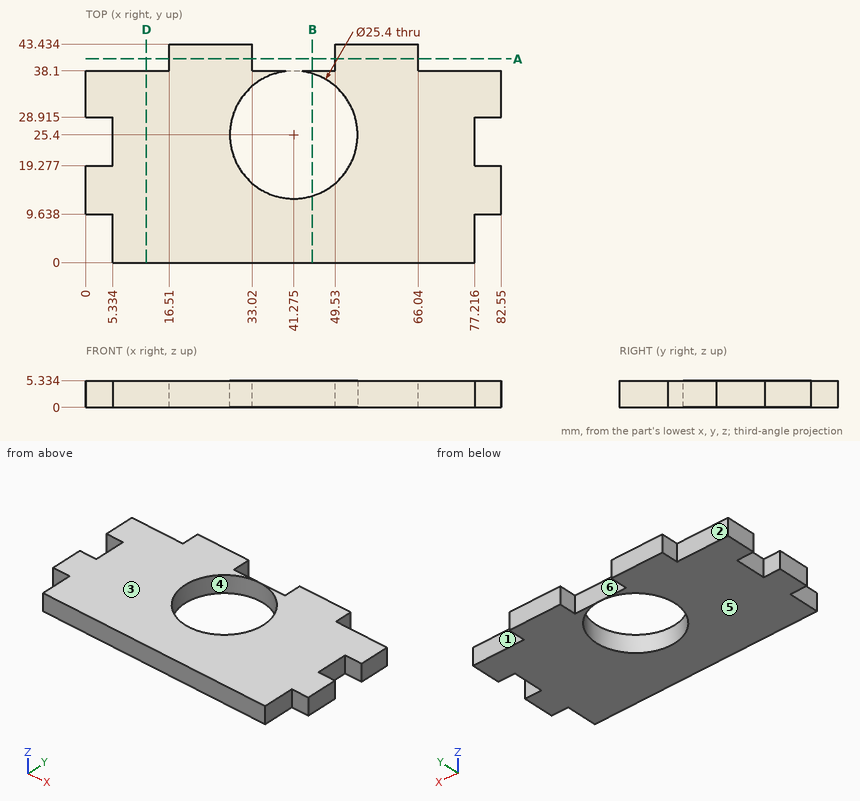
Job drawing, mm, ordinate dimensions from the low corner. One solid piece. A direction names the side the tool comes from. Coordinates: 2 decimals unless noted, no trailing zeros. Order: outer loops, then holes, each group sorted by start corner. A loop starts at its lowest first (then second) coordinate and runs counter-clockwise, first axis right, second up. Notation, with made-up numbers: M 69,87.25 L 92,87.25 A11 ccw 92,107.25 Z; hole C 89.5,10.5 d10. An arc over 180 degrees is marked long. Return JSON: item names as keys, results as strings.
1. Saw through at D-D (x = 12). Give the cut face in (y, z), and give its area (3 significant figures).
Ans:
{"outline": "M 0,0 L 38.1,0 L 38.1,5.33 L 0,5.33 Z", "area": "203 mm^2"}
2. Flat gauge pins, fed straight in: pin 1 (2 mm diameter, centred on y = 23, z = 2.5, fed in from +X); pin 2 (2.5 mm diameter, centred on x = 2, z = 1.5, fed in from +Y); pin 3 (1.6 mm diameter, centred on y = 40.5, z = 2, fed in from +X); pin 4 (15 mm diameter, centred on x = 41.28, y = 25.4, fed in from -Z). Where does each tip first touch, or does it go through?
Ans:
{"pin 1": "x = 77.22", "pin 2": "y = 38.1", "pin 3": "x = 66.04", "pin 4": "through"}
3. Saw through at A-A (y = 40.5). Give the cut face in (x, z), and give its area (3 significant figures).
Ans:
{"outline": "M 16.51,0 L 33.02,0 L 33.02,5.33 L 16.51,5.33 Z; M 49.53,0 L 66.04,0 L 66.04,5.33 L 49.53,5.33 Z", "area": "176 mm^2"}
4. Tool access for the marked faces 1, 2 and 3: list every direction of +Z, -Z, +X, -X, +Y, -Y with a clear straight run to the whole face (end or side of a thin tool).
Ans:
{"face 1": "+Z, -Z, +X, +Y", "face 2": "+Z, -Z, -X, +Y", "face 3": "+Z, +X, -X, +Y, -Y"}
5. Saw through at B-B (x = 45). Give the cut face in (y, z), and give its area (3 significant figures).
Ans:
{"outline": "M 0,0 L 13.26,0 L 13.26,5.33 L 0,5.33 Z; M 37.54,0 L 38.1,0 L 38.1,5.33 L 37.54,5.33 Z", "area": "73.7 mm^2"}
6. Drill centre lines: probe 1 along X at (y, z) = (38.5, 1.95); probe 2 along Y at (x, z) = (6, 1.6); probe 3 along X at (y, z) = (5.5, 3.7). Where is each one in solid material? Low to high.
Ans:
{"probe 1": "16.51 to 33.02, 49.53 to 66.04", "probe 2": "0 to 38.1", "probe 3": "5.33 to 77.22"}
7. Pull direction Y, two halves, no side cores. Call the marked faces 4, 5 and 6: +Y half, -Y half, draft (parallel to the pull), parting line (faces both ways), or undercut.
Ans:
{"face 4": "undercut", "face 5": "draft", "face 6": "+Y half"}
